```python
from build123d import *

# Parameters (mm, degrees)
BOSS_EXTRUDE1_DEPTH = 12.1
SKETCH2_R           = 4
BOSS_EXTRUDE2_DEPTH = 7.17
SKETCH3_R           = 15.9
BOSS_EXTRUDE3_DEPTH = 20
SKETCH4_R           = 3.75
BOSS_EXTRUDE4_DEPTH = 3.2
SKETCH5_R           = 4.5
BOSS_EXTRUDE5_DEPTH = 1.8
BOSS_EXTRUDE6_DEPTH = 5.7
SKETCH8_R           = 6
CUT_EXTRUDE2_DEPTH  = 3
SKETCH7_R           = 1.375
CUT_EXTRUDE1_DEPTH  = 63.607108223
CUT_EXTRUDE3_START  = -1.93
SKETCH9_R           = 6
CUT_EXTRUDE3_DEPTH  = 1.93
FILLET1_R           = 1
FILLET2_R           = 5


with BuildPart() as part:
    # Sketch1 → Boss-Extrude1 (new body)
    with BuildSketch(Plane.XY):
        with BuildLine():
            Line((0, -16.4), (34.4, -16.4))
            ThreePointArc((34.4, -16.4), (46.1, -4.7), (34.4, 7))
            Line((34.4, 7), (14.831048513, 7))
            ThreePointArc((14.831048513, 7), (-13.852075657, 8.779521627), (0, -16.4))
        make_face()
    extrude(amount=BOSS_EXTRUDE1_DEPTH)

    # Sketch2 → Boss-Extrude2 (add)
    with BuildSketch(Plane.XY.offset(9.1)):
        with Locations((17.276313416, 9.163011328)):
            Circle(SKETCH2_R)
        with Locations((46, -12.538367177)):
            Circle(SKETCH2_R)
        with Locations((12.6224468, -15.4)):
            Circle(SKETCH2_R)
    extrude(amount=-BOSS_EXTRUDE2_DEPTH)

    # Sketch3 → Boss-Extrude3 (add)
    with BuildSketch(Plane(origin=(0, 0, 0), x_dir=(-1, 0, 0), z_dir=(0, 0, -1))):
        Circle(SKETCH3_R)
    extrude(amount=BOSS_EXTRUDE3_DEPTH)

    # Sketch4 → Boss-Extrude4 (add)
    with BuildSketch(Plane(origin=(0, 0, -20), x_dir=(-1, 0, 0), z_dir=(0, 0, -1))):
        Circle(SKETCH4_R)
    extrude(amount=BOSS_EXTRUDE4_DEPTH)

    # Sketch5 → Boss-Extrude5 (add)
    with BuildSketch(Plane.XY.offset(12.1)):
        with Locations((34.4, -4.7)):
            Circle(SKETCH5_R)
    extrude(amount=BOSS_EXTRUDE5_DEPTH)

    # Sketch6 → Boss-Extrude6 (add)
    with BuildSketch(Plane.XY.offset(13.9)):
        Polygon((35.996373494, -7.465), (37.592746989, -4.7), (35.996373494, -1.935), (32.803626506, -1.935), (31.207253011, -4.7), (32.803626506, -7.465), align=None)
    extrude(amount=BOSS_EXTRUDE6_DEPTH)

    # Sketch8 → Cut-Extrude2 (cut)
    with BuildSketch(Plane.XY.offset(12.1)):
        with Locations((17.83477741, 12.110572688)):
            Circle(SKETCH8_R)
        with Locations((12.063982807, -18.347561359)):
            Circle(SKETCH8_R)
    extrude(amount=-CUT_EXTRUDE2_DEPTH, mode=Mode.SUBTRACT)

    # Sketch7 → Cut-Extrude1 (cut, through all)
    with BuildSketch(Plane.XY.offset(9.1)):
        with Locations((17.276313416, 9.163011328)):
            Circle(SKETCH7_R)
        with Locations((46, -12.538367177)):
            Circle(SKETCH7_R)
        with Locations((12.6224468, -15.4)):
            Circle(SKETCH7_R)
    extrude(amount=-CUT_EXTRUDE1_DEPTH, mode=Mode.SUBTRACT)

    # Sketch9 → Cut-Extrude3 (cut)
    with BuildSketch(Plane(origin=(0, 0, 0), x_dir=(-1, 0, 0), z_dir=(0, 0, -1)).offset(CUT_EXTRUDE3_START)):
        with Locations((-12.063982807, -18.347561359)):
            Circle(SKETCH9_R)
        with Locations((-17.83477741, 12.110572688)):
            Circle(SKETCH9_R)
    extrude(amount=CUT_EXTRUDE3_DEPTH, mode=Mode.SUBTRACT)

    # Fillet1
    # the kernel refuses this fillet: 1 mm, written as the material it adds along each edge
    with BuildSketch(Plane(origin=(8.749463454, -16.4, 1.93), x_dir=(-1, 0, 0), z_dir=(0, 0, 1))) as fillet1_piece_1:
        with BuildLine():
            CenterArc((0.709592349, 1), FILLET1_R, 203.578178478, 66.421821522)
            ThreePointArc((-0.20692279, 0.6), (-0.091542385, 0.304110525), (0, 0))
            Line((0, 0), (0.709592349, 0))
        make_face()
    extrude(amount=7.17)
    with BuildSketch(Plane(origin=(16.495430147, -16.4, 1.93), x_dir=(1, 0, 0), z_dir=(0, 0, 1))) as fillet1_piece_2:
        with BuildLine():
            CenterArc((0.709592349, -1), FILLET1_R, 90, 66.421821522)
            ThreePointArc((-0.20692279, -0.6), (-0.091542385, -0.304110525), (0, 0))
            Line((0, 0), (0.709592349, 0))
        make_face()
    extrude(amount=7.17)
    with BuildSketch(Plane(origin=(42.116078953, -13.495005719, 9.1), x_dir=(-0.786111356647784, -0.6180848929955987, 0), z_dir=(0, 0, -1))) as fillet1_piece_3:
        with BuildLine():
            CenterArc((1.313089389, -0.998550915), FILLET1_R, 93.084870556, 94.384925022)
            ThreePointArc((0.321575856, -1.128554433), (0.202398335, -0.552420542), (0, 0))
            ThreePointArc((0, 0), (0.629637125, -0.016954289), (1.25927425, 0))
        make_face()
    extrude(amount=7.17)
    with BuildSketch(Plane(origin=(45.438635333, -8.577954356, 9.1), x_dir=(0.2801956563205793, 0.959942911937517, 0), z_dir=(0, 0, -1))) as fillet1_piece_4:
        with BuildLine():
            CenterArc((1.313089389, 0.998550915), FILLET1_R, 172.530204422, 94.384925022)
            ThreePointArc((0.321575856, 1.128554433), (0.202398335, 0.552420542), (0, 0))
            ThreePointArc((0, 0), (0.629637125, 0.016954289), (1.25927425, 0))
        make_face()
    extrude(amount=7.17)
    with BuildSketch(Plane(origin=(13.299776183, 9.595621579, 9.1), x_dir=(-0.6279509963726487, 0.7782528805951172, 0), z_dir=(0, 0, -1))) as fillet1_piece_5:
        with BuildLine():
            CenterArc((1.821464626, 0.998546906), FILLET1_R, 158.597997632, 108.312865848)
            ThreePointArc((0.890421562, 1.363456228), (0.515330012, 0.635935903), (0, 0))
            ThreePointArc((0, 0), (0.88378757, 0.023830743), (1.76757514, 0))
        make_face()
    extrude(amount=7.17)
    with BuildSketch(Plane(origin=(20.641039556, 7, -1.81533395), x_dir=(1, 0, 0), z_dir=(0, 0, 1))) as fillet1_piece_6_section:
        with BuildLine():
            CenterArc((1.49813358, 1), FILLET1_R, 166.549673426, 103.450326574)
            ThreePointArc((0.525561636, 1.232602266), (0.314762115, 0.59413715), (0, 0))
            Line((0, 0), (1.49813358, 0))
        make_face()
    fillet1_piece_6 = extrude(amount=10.91533395, mode=Mode.PRIVATE)
    fillet1_piece_6 = fillet1_piece_6 - Plane(origin=(17.83477741, 12.110572688, 0.965), x_dir=(-1, 0, 0), z_dir=(0, 0, 1)) * Cylinder(6, 28, mode=Mode.PRIVATE)
    fillet1_piece_6 = split(fillet1_piece_6, bisect_by=Plane(origin=(21.45614867, 7.07760615, 0), z_dir=(0, 0, 1)), keep=Keep.TOP, mode=Mode.PRIVATE)
    fillet1_piece_6 = split(fillet1_piece_6, bisect_by=Plane(origin=(21.45614867, 7.07760615, 1.93), z_dir=(0, 0, -1)), keep=Keep.TOP, mode=Mode.PRIVATE)
    add(fillet1_piece_6)
    with BuildSketch(Plane(origin=(20.641039556, 7, 1.93), x_dir=(1, 0, 0), z_dir=(0, 0, 1))) as fillet1_piece_7_section:
        with BuildLine():
            CenterArc((1.49813358, 1), FILLET1_R, 166.549673426, 103.450326574)
            ThreePointArc((0.525561636, 1.232602266), (0.314762115, 0.59413715), (0, 0))
            Line((0, 0), (1.49813358, 0))
        make_face()
    fillet1_piece_7 = extrude(amount=7.17, mode=Mode.PRIVATE)
    fillet1_piece_7 = fillet1_piece_7 - Plane(origin=(17.83477741, 12.110572688, 5.515), x_dir=(-1, 0, 0), z_dir=(0, 0, 1)) * Cylinder(6, 21, mode=Mode.PRIVATE)
    add(fillet1_piece_7)
    with BuildSketch(Plane(origin=(20.641039556, 7, 1.93), x_dir=(1, 0, 0), z_dir=(0, 0, 1))) as fillet1_piece_8_section:
        with BuildLine():
            CenterArc((1.49813358, 1), FILLET1_R, 166.549673426, 103.450326574)
            ThreePointArc((0.525561636, 1.232602266), (0.314762115, 0.59413715), (0, 0))
            Line((0, 0), (1.49813358, 0))
        make_face()
    fillet1_piece_8 = extrude(amount=7.17, mode=Mode.PRIVATE)
    fillet1_piece_8 = fillet1_piece_8 & Plane(origin=(17.83477741, 12.110572688, 5.515), x_dir=(-1, 0, 0), z_dir=(0, 0, 1)) * Cylinder(6, 21, mode=Mode.PRIVATE)
    add(fillet1_piece_8)
    with BuildSketch(Plane(origin=(20.641039556, 7, 1.93), x_dir=(1, 0, 0), z_dir=(0, 0, 1))) as fillet1_piece_9_section:
        with BuildLine():
            CenterArc((1.49813358, 1), FILLET1_R, 166.549673426, 103.450326574)
            ThreePointArc((0.525561636, 1.232602266), (0.314762115, 0.59413715), (0, 0))
            Line((0, 0), (1.49813358, 0))
        make_face()
    fillet1_piece_9 = extrude(amount=10.91533395, mode=Mode.PRIVATE)
    fillet1_piece_9 = fillet1_piece_9 - Plane(origin=(17.83477741, 12.110572688, 10.6), x_dir=(-1, 0, 0), z_dir=(0, 0, 1)) * Cylinder(6, 28, mode=Mode.PRIVATE)
    fillet1_piece_9 = split(fillet1_piece_9, bisect_by=Plane(origin=(21.45614867, 7.07760615, 9.1), z_dir=(0, 0, 1)), keep=Keep.TOP, mode=Mode.PRIVATE)
    fillet1_piece_9 = split(fillet1_piece_9, bisect_by=Plane(origin=(21.45614867, 7.07760615, 12.1), z_dir=(0, 0, -1)), keep=Keep.TOP, mode=Mode.PRIVATE)
    add(fillet1_piece_9)

    # Fillet2
    # the kernel refuses this fillet: 5 mm, written as the material it takes off along each edge
    with BuildSketch(Plane(origin=(17.739104369, -16.4, -7.132871381), x_dir=(-0.4856410354617555, 0.8741583292948903, 0), z_dir=(0, 0, 1))) as fillet2_piece_1:
        with BuildLine():
            CenterArc((2.985185629, -4.922308749), FILLET2_R, 100.113527083, 50.831993071)
            Line((-1.385606017, -2.494103572), (0, 0))
            ThreePointArc((0, 0), (1.053594928, -0.093229501), (2.107189856, 0))
        make_face()
    extrude(amount=9.062871381, mode=Mode.SUBTRACT)
    with BuildSketch(Plane(origin=(6.388861244, -16.4, -7.132871381), x_dir=(-1, 0, 0), z_dir=(0, 0, 1))) as fillet2_piece_2:
        with BuildLine():
            CenterArc((2.853148552, -5), FILLET2_R, 90, 50.831993071)
            ThreePointArc((-1.023337864, -1.842017564), (-0.430171587, -0.966284853), (0, 0))
            Line((0, 0), (2.853148552, 0))
        make_face()
    extrude(amount=9.062871381, mode=Mode.SUBTRACT)
    with BuildSketch(Plane(origin=(17.739104369, -16.4, 9.1), x_dir=(-0.4856410354617568, 0.8741583292948896, 0), z_dir=(0, 0, 1))) as fillet2_piece_3:
        with BuildLine():
            CenterArc((2.985185629, -4.922308749), FILLET2_R, 100.113527083, 50.831993071)
            Line((-1.385606017, -2.494103572), (0, 0))
            ThreePointArc((0, 0), (1.053594928, -0.093229501), (2.107189856, 0))
        make_face()
    extrude(amount=10.132871381, mode=Mode.SUBTRACT)
    with BuildSketch(Plane(origin=(6.388861244, -16.4, 9.1), x_dir=(-1, 0, 0), z_dir=(0, 0, 1))) as fillet2_piece_4:
        with BuildLine():
            CenterArc((2.853148552, -5), FILLET2_R, 90, 50.831993071)
            ThreePointArc((-1.023337864, -1.842017564), (-0.430171587, -0.966284853), (0, 0))
            Line((0, 0), (2.853148552, 0))
        make_face()
    extrude(amount=10.132871381, mode=Mode.SUBTRACT)
    with BuildSketch(Plane(origin=(11.890467167, 11.294989621, 1.93), x_dir=(-0.7264583233980587, 0.6872105240504408, 0), z_dir=(0, 0, -1))) as fillet2_piece_5:
        with BuildLine():
            CenterArc((1.484745631, -4.99286384), FILLET2_R, 86.938483712, 31.524868326)
            ThreePointArc((-0.898237104, -0.597253156), (-0.435669612, -0.318853072), (0, 0))
            ThreePointArc((0, 0), (0.875893106, 0.023406604), (1.751786212, 0))
        make_face()
    extrude(amount=1.93, mode=Mode.SUBTRACT)
    with BuildSketch(Plane(origin=(21.423177854, 7.301894881, -3.534616353), x_dir=(0.9267551866460263, -0.37566584090743305, 0), z_dir=(0, 0, 1))) as fillet2_piece_6:
        with BuildLine():
            CenterArc((2.681955321, -4.633775933), FILLET2_R, 112.065471844, 23.198889906)
            Line((-0.869853786, -1.114592496), (-1.225034697, -0.762674153))
            ThreePointArc((-1.225034697, -0.762674153), (-0.796151939, -0.275387861), (-0.427668726, 0.259035636))
            Line((-0.427668726, 0.259035636), (0.200649047, 0.457973755))
            ThreePointArc((0.200649047, 0.457973755), (0.589131014, 0.452569916), (0.615793196, 0.463377593))
            Line((0.615793196, 0.463377593), (0.803626117, 0))
        make_face()
    extrude(amount=5.464616353, mode=Mode.SUBTRACT)
    with BuildSketch(Plane(origin=(21.423177854, 7.301894881, 15.634616353), x_dir=(0.9267551866460257, -0.3756658409074346, 0), z_dir=(0, 0, -1))) as fillet2_piece_7:
        with BuildLine():
            CenterArc((2.681955321, 4.633775933), FILLET2_R, 224.73563825, 23.198889906)
            Line((-0.869853786, 1.114592496), (-1.225034697, 0.762674153))
            ThreePointArc((-1.225034697, 0.762674153), (-0.796151939, 0.275387861), (-0.427668726, -0.259035636))
            Line((-0.427668726, -0.259035636), (0.200649047, -0.457973755))
            ThreePointArc((0.200649047, -0.457973755), (0.589131014, -0.452569916), (0.615793196, -0.463377593))
            Line((0.615793196, -0.463377593), (0.803626117, 0))
        make_face()
    extrude(amount=6.534616353, mode=Mode.SUBTRACT)
    with BuildSketch(Plane(origin=(11.890467167, 11.294989621, 16.479465531), x_dir=(-0.7264583233980683, 0.6872105240504307, 0), z_dir=(0, 0, -1))) as fillet2_piece_8:
        with BuildLine():
            CenterArc((1.484745631, -4.99286384), FILLET2_R, 86.938483712, 31.524868326)
            ThreePointArc((-0.898237104, -0.597253156), (-0.435669612, -0.318853072), (0, 0))
            ThreePointArc((0, 0), (0.875893106, 0.023406604), (1.751786212, 0))
        make_face()
    extrude(amount=7.379465531, mode=Mode.SUBTRACT)


solid = part.part
```
Source: CAD feature listing. Evaluate the final solid. Frame: model axes, mm. A direction names the side the tool comes from. Give positions to 0.01 mm unless a question says otherwise; leave off trailing zeros. Order: outer loops, then holes, each group sorted by start corner. A loop starts at its lowest first (then second) coordinate and runs counter-clockwise, first axis right, second up.
(1) Section query C-C (x = -9). Return the cut outline in (y, z), plus the area to 3 significant figures.
(2) Contact query for flat-ended pins moving along their axis: P1, Ø10, axis at x = 22.5, y = -5.5, coming from the -Z side; P2, Ø6, axis at x = 12.5, y = 7, coming from the -Z side; P3, Ø3, axis at x = 17.28, y = 9.16, coming from the +Z side. Output: stop coordinate, or through.
(3) Pull-direction query (Y, two-part tool) for faces 1 (the face through (34, -1.935, 17)), 2 (the face through (44.626, -12.478, 5.565)), 3 (the face through (0, 0, -23.2)), 4 (the face through (18.418, -15.903, 10.579)); classes: +Y half, -Y half, draft (parallel to the pull), parting line (faces both ways), or undercut.
(4) Section query B-B (z = -15.5). Return the cut outline in (x, y), plus the area to 3 significant figures.
(5) Access query for faces 5 (the face through (12, -17, 9.1)), 6 (the face through (36.806, -3.337, 16.71)), 7 (the face through (31.994, -6.063, 16.71)), 8 (the face through (3.746, 0.165, -21.578)). Directions: +Z, -Z, +X, -X, +Y, -Y. A direction counts if a zero-diameter tool reaches every point of the face in a straight line with its end or side. Return the directions, or none.
(6) Material intervals for line 1 along Z through (x, y) = (30, -11.5); line 2 along Y through (x, z) = (32.5, 4); line 3 along Z through (x, y) = (7, -10), sorted ascending.
(7) Section query D-D (y = -3). Return the cut outline in (x, z).
(8) Section query A-A (y = 5). Return the cut outline in (x, z), plus the area to 3 significant figures.
Outcome:
1. outline: (-13.71, 0) - (-13.11, 0) - (-13.11, -20) - (13.11, -20) - (13.11, 0) - (13.71, 0) - (13.71, 12.1) - (-13.71, 12.1) - close
1. area: 856 mm2
2. P1: stops at z = 0
2. P2: stops at z = -20
2. P3: stops at z = 9.1
3. face 1: +Y half
3. face 2: undercut
3. face 3: draft
3. face 4: -Y half
4. outline: circle Ø31.8 at (0, 0)
4. area: 794 mm2
5. face 5: +Z, -Y
5. face 6: +Z, +X, +Y
5. face 7: +Z, -X, -Y
5. face 8: -Z
6. line 1: z = 0 to 12.1
6. line 2: y = -16.4 to 7
6. line 3: z = -20 to 12.1
7. outline: (-16.12, 0) - (-15.61, 0) - (-15.61, -20) - (-2.25, -20) - (-2.25, -23.2) - (2.25, -23.2) - (2.25, -20) - (15.61, -20) - (15.61, 0) - (45.98, 0) - (45.98, 12.1) - (38.57, 12.1) - (38.57, 13.9) - (36.61, 13.9) - (36.61, 19.6) - (32.19, 19.6) - (32.19, 13.9) - (30.23, 13.9) - (30.23, 12.1) - (-16.12, 12.1) - close
8. outline: (-15.62, 0) - (-15.09, 0) - (-15.09, -20) - (15.09, -20) - (15.09, 0) - (40.94, 0) - (40.94, 12.1) - (-15.62, 12.1) - close
8. area: 1,290 mm2
